Geometry check sheet. Reference: drawing and pictorial views, mm from the part's lowest x, y, z. A direction names the side the tool comes from. Coordinates: 2 decimals unless noted, no trailing zeros. Loops run counter-clockwise (first coordinate to the right, second up) from the corner with the lowest first, then second, coordinate; pieces in that order, holes last. Notation, with made-up numbers: (66.25, 43.5) - (77.25, 43.5) arc R15 cw to (77.25, 69.5) - close; hole circle Ø3 at (44.5, 33.5). An arc over 180 degrees is marked (long way). One line per item, written item: value.
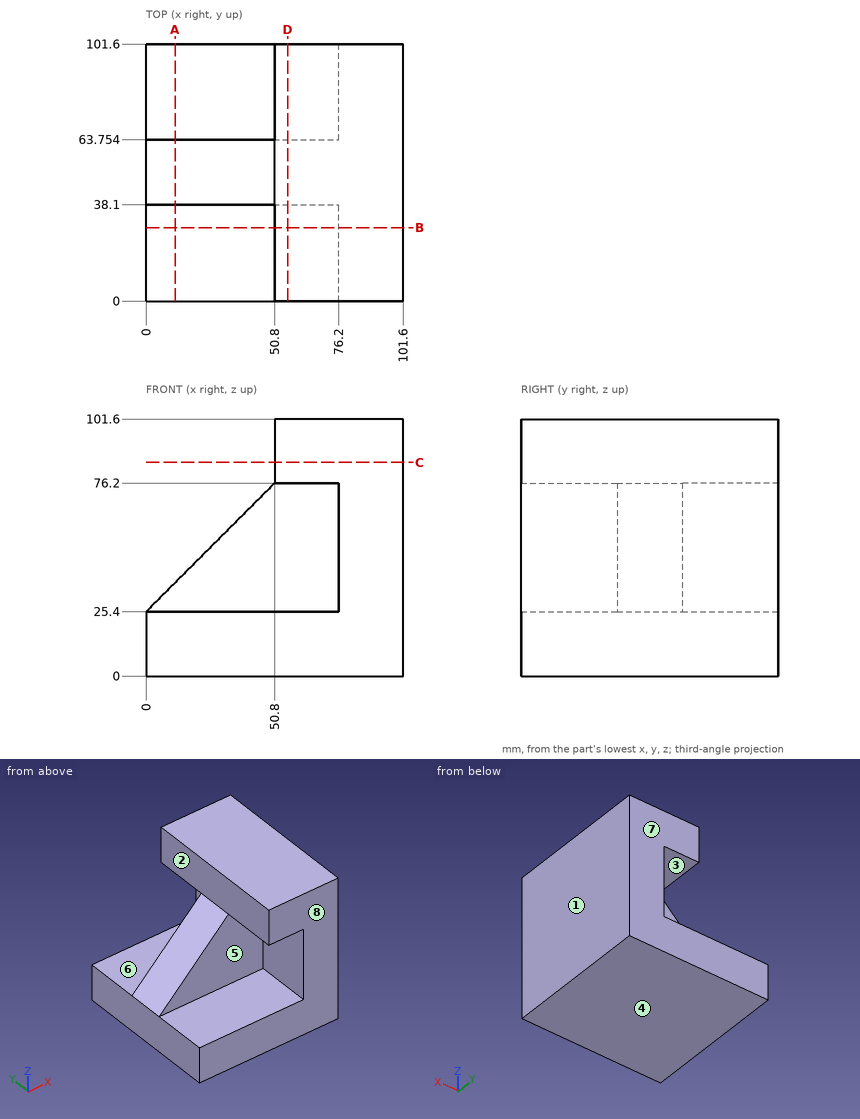
(1) Cross-section at A-A on x = 11.5. Record the cut outline in (y, z), and give its area (3 significant figures).
Reply:
outline: (0, 0) - (101.6, 0) - (101.6, 25.4) - (63.75, 25.4) - (63.75, 36.9) - (38.1, 36.9) - (38.1, 25.4) - (0, 25.4) - close
area: 2,880 mm2
(2) Cross-section at B-B on y = 29. Record the cut outline in (x, z).
Reply:
outline: (0, 0) - (101.6, 0) - (101.6, 101.6) - (50.8, 101.6) - (50.8, 76.2) - (76.2, 76.2) - (76.2, 25.4) - (0, 25.4) - close
(3) Access from +Z, -Z, +X, -X, +Y, -Y to the whole of each face (thin tool, end or side, straight path). Record for the marked faces 1, 2, 3, 4 and 5.
Reply:
face 1: +Z, -Z, +X, +Y, -Y
face 2: +Z, -X, +Y, -Y
face 3: -X, +Y
face 4: -Z, +X, -X, +Y, -Y
face 5: -X, -Y
(4) Release check for a two-part mould opening along Y. For the marked faces 6, 7 and 8 record: pulls with the +Y half, pulls with the -Y half, needs draft (parallel to the pull), parting line crosses it, or undercut.
Reply:
face 6: needs draft
face 7: pulls with the +Y half
face 8: pulls with the -Y half
(5) Material ranges on probe 1 along Z at (x, y) = (72.5, 91.5); probe 2 along Y at (x, z) = (28, 29); probe 3 along X at (y, z) = (50, 77), recorded low to high. Write a range as from..to.
Reply:
probe 1: 0..25.4, 76.2..101.6
probe 2: 38.1..63.75
probe 3: 50.8..101.6
(6) Cross-section at D-D on x = 56. Record the cut outline in (y, z).
Reply:
outline: (0, 0) - (101.6, 0) - (101.6, 25.4) - (63.75, 25.4) - (63.75, 76.2) - (101.6, 76.2) - (101.6, 101.6) - (0, 101.6) - (0, 76.2) - (38.1, 76.2) - (38.1, 25.4) - (0, 25.4) - close
(7) Cross-section at C-C on z = 84.5. Record the cut outline in (x, y).
Reply:
outline: (50.8, 0) - (101.6, 0) - (101.6, 101.6) - (50.8, 101.6) - close
(8) Go/stop test with flat-tipped pins: pin 1 Ø12 at (y, z) = (43, 80.5) entering from -X; pin 2 Ø2 at (y, z) = (54.5, 78.5) entering from -X; pin 3 Ø4 at (x, z) = (42, 29) entering from -Y. Record where each tip stops, or that it passes through.
Reply:
pin 1: x = 49.1
pin 2: x = 50.8
pin 3: y = 38.1
